For this review, take the finished solid that the model builds, in its own axes (mm). Face numbers are marked on the shaded views. A direction names the side the tool comes from. Give positions to 0.01 mm unless a question says otherwise; leave off trailing zeros. Loops run counter-clockwise (first coordinate to the right, second up) from the corner with the lowest first, then second, coordinate; pieces in that order, holes last.
Autodesk Inventor part; units mm, degrees
ref_plane "YZ Plane" through (0, 0, 0) normal (1, 0, 0) x (0, 1, 0)
ref_plane "XZ Plane" through (0, 0, 0) normal (0, 1, 0) x (-1, 0, 0)
ref_plane "XY Plane" through (0, 0, 0) normal (0, 0, 1) x (1, 0, 0)
sketch "Sketch1" plane through (0, 0, 0) normal (0, 0, 1) x (1, 0, 0)
  circle A0 centre (0.8326, 3.0356) radius 2.5
  point P0 (0, 0)
  dimension "d0" = 5
extrude "Extrusion1" add sketch "Sketch1" along normal blind 29.972
sketch "Sketch2" plane through (0.8326, 3.0356, 29.972) normal (0, 0, 1) x (1, 0, 0)
  circle A0 centre (0, 0) radius 2.5
  circle A1 centre (0, 0) radius 5.015
  point P0 (-0.8326, -3.0356)
extrude "Extrusion2" add sketch "Sketch2" along normal blind 7.5 contours A0 | A1
sketch "Sketch3" plane through (0.8326, 3.0356, 0) normal (0, 0, -1) x (-1, 0, 0)
  circle A0 centre (0, 0) radius 5.015
  circle A1 centre (0, 0) radius 2.5
  circle A2 centre (0, 0) radius 2.5
  point P0 (0.8326, -3.0356)
extrude "Extrusion3" add sketch "Sketch3" along normal blind 6 contours A1
sketch "Sketch4" plane through (0.8326, 3.0356, -6) normal (0, 0, -1) x (-1, 0, 0)
  circle A0 centre (0, 0) radius 2.5
  point P0 (0.8326, -3.0356)
extrude "Extrusion4" cut sketch "Sketch4" against normal blind 19.05
properties part number "5mm_bolt_short" material "Steel, Alloy"
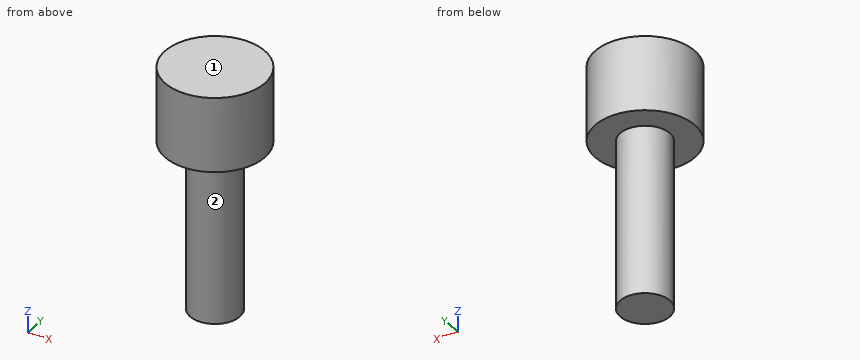
Item 1: Take a section at C-C on z = 16.5. Give the boundary of the cut face in (x, y).
Answer:
outline: circle Ø5 at (0.83, 3.04)
Item 2: Take a section at B-B on x = -1.25. Give the boundary of the cut face in (y, z), and give its area (3 significant figures).
Answer:
outline: (-1.53, 29.97) - (1.65, 29.97) - (1.65, 13.05) - (4.42, 13.05) - (4.42, 29.97) - (7.6, 29.97) - (7.6, 37.47) - (-1.53, 37.47) - close
area: 115 mm2
Item 3: Take a section at A-A on y = 3.5. Give the boundary of the cut face in (x, z), and give its area (3 significant figures).
Answer:
outline: (-4.16, 29.97) - (-1.62, 29.97) - (-1.62, 13.05) - (3.29, 13.05) - (3.29, 29.97) - (5.83, 29.97) - (5.83, 37.47) - (-4.16, 37.47) - close
area: 158 mm2
Item 4: Clearance check with flat-ended pins moving along their axes: pin 1 Ø5 at (y, z) = (6, 23.5) entering from +X; pin 2 Ø5 at (y, z) = (2.5, 23.5) entering from -X; pin 3 Ø2 at (y, z) = (5.5, 20.5) entering from +X. State where each tip first meets the part, or that it passes through.
Answer:
pin 1: stops at x = 3.29
pin 2: stops at x = -1.67
pin 3: stops at x = 2.86
Item 5: For L1, parallel to Y at x = 1, z = 23.25; L2, parallel to Z at x = -1, y = 1; L3, parallel to X at y = 3.5, z = 22.75, list the stretches that pass through material, from the lowest coordinate up.
Answer:
L1: y = 0.54 to 5.53
L2: z = 29.97 to 37.47
L3: x = -1.62 to 3.29
Item 6: Take a section at D-D on y = 7.25. Give the boundary of the cut face in (x, z).
Answer:
outline: (-1.89, 29.97) - (3.55, 29.97) - (3.55, 37.47) - (-1.89, 37.47) - close
Item 7: Tool access review of the marked faces 1 and 2: name each direction out of +Z, -Z, +X, -X, +Y, -Y from which nothing blocks a thin tool from reaching the whole face with its end or side.
Answer:
face 1: +Z, +X, -X, +Y, -Y
face 2: -Z
